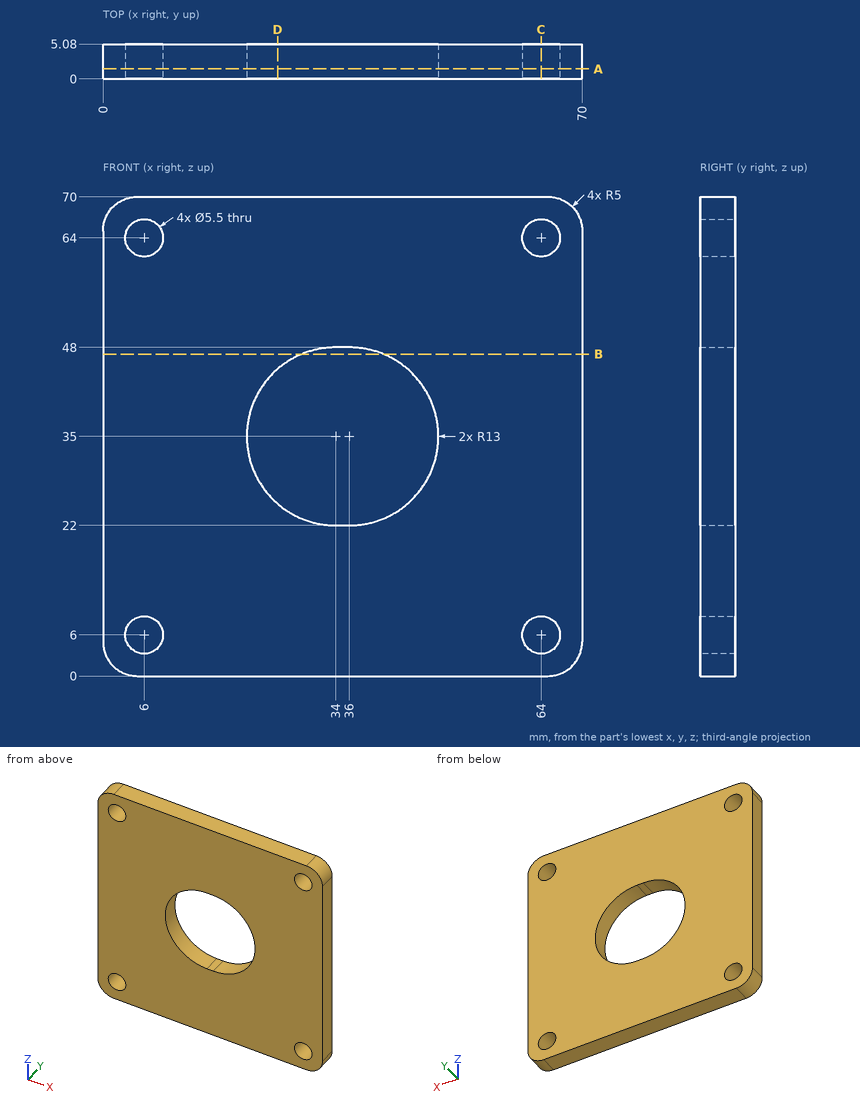
Input: dimensioned drawing with shaded views. Units: mm. Origin: part minimum x, y, z. Coordinates: 2 decimals unless noted, no trailing zeros. Loops run counter-clockwise (first coordinate to the right, second up) from the corner with the lowest first, then second, coordinate; pieces in that order, holes last.
Q1. Section B-B, the plane z = 47. Return the cut outline in (x, y), and give its area (3 significant figures).
Results are:
outline: (0, 0) - (29, 0) - (29, 5.08) - (0, 5.08) - close; (41, 0) - (70, 0) - (70, 5.08) - (41, 5.08) - close
area: 295 mm2
Q2. Section A-A, the plane y = 1.45. Return the cut outline in (x, z), and give its area (3 significant figures).
Results are:
outline: (0, 5) arc R5 ccw to (5, 0) - (65, 0) arc R5 ccw to (70, 5) - (70, 65) arc R5 ccw to (65, 70) - (5, 70) arc R5 ccw to (0, 65) - close; hole circle Ø5.5 at (6, 6); hole circle Ø5.5 at (6, 64); hole (34, 22) - (36, 22) arc R13 ccw to (36, 48) - (34, 48) arc R13 ccw to start; hole circle Ø5.5 at (64, 6); hole circle Ø5.5 at (64, 64)
area: 4,200 mm2
Q3. Contact query for flat-ended pins moving along their axis: pin 1 (7 mm diameter, centred on x = 6, z = 6, fed in from +Y); pin 2 (3.5 mm diameter, centred on x = 64, z = 6, fed in from +Y). Output: stop coordinate, or through.
Results are:
pin 1: stops at y = 5.08
pin 2: passes through
Q4. Section D-D, the plane x = 25.5. Return the cut outline in (y, z).
Results are:
outline: (0, 0) - (5.08, 0) - (5.08, 25.16) - (0, 25.16) - close; (0, 44.84) - (5.08, 44.84) - (5.08, 70) - (0, 70) - close
Q5. Section C-C, the plane x = 64. Return the cut outline in (y, z), and give its area (3 significant figures).
Results are:
outline: (0, 0) - (5.08, 0) - (5.08, 3.25) - (0, 3.25) - close; (0, 8.75) - (5.08, 8.75) - (5.08, 61.25) - (0, 61.25) - close; (0, 66.75) - (5.08, 66.75) - (5.08, 70) - (0, 70) - close
area: 300 mm2
Q6. Line query: line 1 along X through (y, z) = (3.4, 6); line 2 along X through (y, z) = (2.35, 30); line 3 along Z through (x, y) = (7.5, 0.8). Output: solid intervals per line, ascending.
Results are:
line 1: x = 0 to 3.25, 8.75 to 61.25, 66.75 to 70
line 2: x = 0 to 22, 48 to 70
line 3: z = 0 to 3.7, 8.3 to 61.7, 66.3 to 70
